Read the model definition and answer for the solid it produces. Units are mm, in the model's axes. A direction names the side the tool comes from. Give positions to 0.01 mm unless a question says otherwise; leave off trailing zeros. Loops run counter-clockwise (first coordinate to the right, second up) from the corner with the lowest first, then second, coordinate; pieces in that order, holes last.
(1) Find section C-C, the plane z = -9. Write down the section's boundary in (x, y).
(2) Find section D-D, the plane z = -24. Write down the section's boundary in (x, y), then the cut area to 3 significant figures.
(3) Find section B-B, the plane x = 36. Write down the section's boundary in (y, z), then the cut area to 3 significant figures.
(4) Determine the mould class of faces 4 (the face through (86, 5, -16)), 5 (the face through (0, 32, -32)), 6 (the face through (86, 5, -32)), 7 (the face through (36, 21, -22)) for opening direction Z: pulls with the +Z half, pulls with the -Z half, needs draft (parallel to the pull), parting line crosses it, or undercut.
(5) Straight lines are drawn through the part: probe 1 along Z at (x, y) = (83, 8); probe 2 along X at (y, z) = (24, -61); probe 3 along X at (y, z) = (39.5, -51). For each, find the intervals that lie inside material, in ascending order.
(6) Find section A-A, the plane y = 8.5. Write down the section's boundary in (x, z).
(7) Each of these flat-tipped pins is pushed along its axis until it touches: P1, Ø12, axis at x = 24.5, y = 20.5, coming from the +Z side; P2, Ø22.5, axis at y = 28.5, z = -30, coming from the +X side; P3, Ø8, axis at x = 29.5, z = -32.5, coming from the -Y side; P4, Ø2.5, axis at x = 53.5, z = -50.5, coming from the +Y side. Where does it stop, or does it pass through?
(8) Which of the six approach directions +Z, -Z, +X, -X, +Y, -Y give full straight-line access (tool end or side, diameter ignored) to faces 1 (the face through (8, 64, -56)), 2 (the face through (56, 24, -37)), 3 (the face through (52, 38, -43))?
```python
from build123d import *

# Parameters (mm, degrees)
SKETCH2_W           = 96
SKETCH2_H           = 64
BOSS_EXTRUDE1_DEPTH = 10
CUT_EXTRUDE3_DEPTH  = 13
BOSS_EXTRUDE4_DEPTH = 16
SKETCH8_W           = 40
SKETCH8_H           = 42
BOSS_EXTRUDE6_DEPTH = 28
CUT_EXTRUDE4_REACH  = 124.784
SKETCH9_R           = 12
BOSS_EXTRUDE7_DEPTH = 12


with BuildPart() as part:
    # Sketch2 → Boss-Extrude1 (new body)
    with BuildSketch(Plane(origin=(0, 0, 0), x_dir=(1, 0, 0), z_dir=(0, 1, 0))):
        with Locations((48, 32)):
            Rectangle(SKETCH2_W, SKETCH2_H)
    extrude(amount=BOSS_EXTRUDE1_DEPTH)

    # Sketch3 → Cut-Extrude3 (cut)
    with BuildSketch(Plane(origin=(0, 10, 0), x_dir=(1, 0, 0), z_dir=(0, 1, 0))):
        with BuildLine():
            Line((96, 16), (76, 16))
            ThreePointArc((76, 16), (68, 24), (76, 32))
            Line((76, 32), (96, 32))
            ThreePointArc((96, 32), (104, 24), (96, 16))
        make_face()
    extrude(amount=-CUT_EXTRUDE3_DEPTH, mode=Mode.SUBTRACT)

    # Sketch7 → Boss-Extrude4 (add)
    with BuildSketch(Plane.ZY):
        with BuildLine():
            Line((-64, 0), (0, 0))
            Line((0, 0), (0, 16))
            ThreePointArc((0, 16), (-14.058874503, 49.941125497), (-48, 64))
            Line((-48, 64), (-64, 64))
            Line((-64, 64), (-64, 0))
        make_face()
    extrude(amount=-BOSS_EXTRUDE4_DEPTH)

    # Sketch8 → Boss-Extrude6 (add)
    with BuildSketch(Plane(origin=(0, 10, 0), x_dir=(1, 0, 0), z_dir=(0, 1, 0))):
        with Locations((36, 43)):
            Rectangle(SKETCH8_W, SKETCH8_H)
    extrude(amount=BOSS_EXTRUDE6_DEPTH)

    # Sketch9 → Cut-Extrude4 (cut, up to next)
    with BuildSketch(Plane.XY.offset(-22), mode=Mode.PRIVATE) as cut_extrude4_sk1:
        with Locations((36, 38)):
            Circle(SKETCH9_R)
    cut_extrude4_tool1 = extrude(cut_extrude4_sk1.sketch, amount=-CUT_EXTRUDE4_REACH, mode=Mode.PRIVATE) & part.part
    add(cut_extrude4_tool1.solids().sort_by_distance((36, 38, -22))[0], mode=Mode.SUBTRACT)

    # Sketch15 → Boss-Extrude7 (add)
    with BuildSketch(Plane(origin=(0, 0, -64), x_dir=(-1, 0, 0), z_dir=(0, 0, -1))):
        Polygon((-96, 10), (-56, 38), (-56, 10), align=None)
    extrude(amount=-BOSS_EXTRUDE7_DEPTH)


solid = part.part
```
Entries:
1. outline: (0, 0) - (96, 0) - (96, 10) - (16, 10) - (16, 43.98) - (0, 43.98) - close
2. outline: (0, 0) - (68, 0) - (68, 10) - (56, 10) - (56, 38) - (48, 38) arc R12 cw to (24, 38) - (16, 38) - (16, 57.57) - (0, 57.57) - close
2. area: 2,330 mm2
3. outline: (0, -64) - (26, -64) - (26, -22) - (10, -22) - (10, 0) - (0, 0) - close
3. area: 1,310 mm2
4. face 4: undercut
4. face 5: needs draft
4. face 6: undercut
4. face 7: pulls with the +Z half
5. probe 1: z = -64 to -32, -16 to 0
5. probe 2: x = 0 to 76
5. probe 3: x = 0 to 16
6. outline: (0, -64) - (96, -64) - (96, -32) - (76, -32) arc R8 cw to (76, -16) - (96, -16) - (96, 0) - (0, 0) - close
7. P1: stops at z = -22
7. P2: stops at x = 56
7. P3: stops at y = 0
7. P4: stops at y = 38
8. face 1: +Z, -Z, +X, -X, +Y
8. face 2: +Z, +X, +Y
8. face 3: +Z, -Z, +X, +Y
